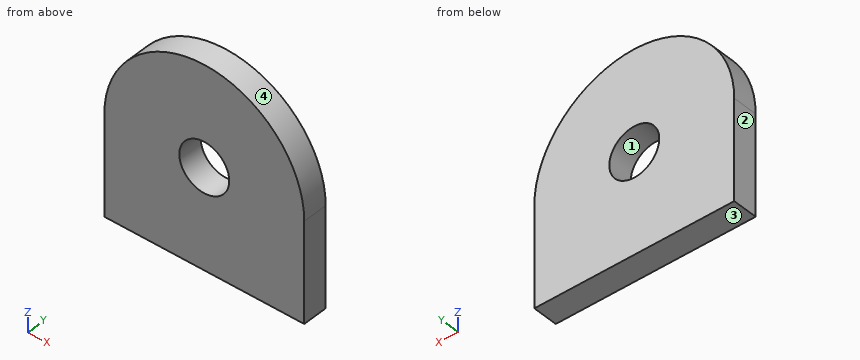
```python
from build123d import *

# Parameters (mm, degrees)
F0_R     = 12.7
F1_DEPTH = 12.7


with BuildPart() as f1:
    # F0 (on Front) → F1 (new body)
    with BuildSketch(Plane.XZ):
        with BuildLine():
            ThreePointArc((50.8, 0), (0, 50.8), (-50.8, 0))
            Line((-50.8, 0), (-50.8, -50.8))
            Line((-50.8, -50.8), (50.8, -50.8))
            Line((50.8, -50.8), (50.8, 0))
        make_face()
        Circle(F0_R, mode=Mode.SUBTRACT)
    extrude(amount=F1_DEPTH)


solid = f1.part
```
The listing builds one solid part. Answer for the finished solid, in the listing's coordinates (mm). Face numbers are marked on the shaded views. Round coordinates to 2 decimals unless told otherwise and drop trailing zeros. Loops run counter-clockwise (first coordinate to the right, second up) from the corner with the lowest first, then second, coordinate; pieces in that order, holes last.
Q1. For a pull along X with two mould halves and no side action, classify the marked faces 1, 2, 3 and 4 as released by +X, released by -X, zero draft, split by the parting line, or undercut.
Q2. Section A-A, the plane x = 0 is taken. Determine the outline of the cut face in (y, z).
Q3. Section D-D, the plane x = 29.5 is taken. Determine the outline of the cut face in (y, z).
Q4. Section C-C, the plane y = -4 is taken. Determine the outline of the cut face in (x, z), then the cut area to 3 significant figures.
Q5. Find the intervals of material crossed by line 1 (Z direction, x = 0, y = -10); line 2 (Z direction, x = -5, y = -5.5); line 3 (X direction, y = -3.5, z = -4), in increasing order.
Q6. Given pin 1 Ø6 at (x, y) = (28, -5) entering from +Z; pin 2 Ø1.5 at (y, z) = (-10.5, 13) entering from -X; pin 3 Ø4 at (y, z) = (-5.5, 23.5) entering from +X, each flat-ended and moving along its own axis, determine where each tip first touches the part or whether it passes through.
Q7. Section B-B, the plane z = -9 is taken. Determine the outline of the cut face in (x, y), then the cut area to 3 significant figures.
Completed:
1. face 1: undercut
1. face 2: released by -X
1. face 3: zero draft
1. face 4: split by the parting line
2. outline: (-12.7, -50.8) - (0, -50.8) - (0, -12.7) - (-12.7, -12.7) - close; (-12.7, 12.7) - (0, 12.7) - (0, 50.8) - (-12.7, 50.8) - close
3. outline: (-12.7, -50.8) - (0, -50.8) - (0, 41.36) - (-12.7, 41.36) - close
4. outline: (-50.8, -50.8) - (50.8, -50.8) - (50.8, 0) arc R50.8 ccw to (-50.8, 0) - close; hole circle Ø25.4 at (0, 0)
4. area: 8,710 mm2
5. line 1: z = -50.8 to -12.7, 12.7 to 50.8
5. line 2: z = -50.8 to -11.67, 11.67 to 50.55
5. line 3: x = -50.8 to -12.05, 12.05 to 50.8
6. pin 1: stops at z = 44.22
6. pin 2: stops at x = -49.3
6. pin 3: stops at x = 46.03
7. outline: (-50.8, -12.7) - (-8.96, -12.7) - (-8.96, 0) - (-50.8, 0) - close; (8.96, -12.7) - (50.8, -12.7) - (50.8, 0) - (8.96, 0) - close
7. area: 1,060 mm2
